Input: dimensioned drawing with shaded views. Units: mm. Origin: part minimum x, y, z. A direction names the side the tool comes from. Coordinates: 2 decimals unless noted, no trailing zeros. Loops run counter-clockwise (first coordinate to the right, second up) from the corner with the lowest first, then second, coordinate; pieces in that order, holes last. Notation, with made-up numbers: (-13, 32.5) - (36, 32.5) arc R17 cw to (36, 61.5) - close; hole circle Ø11 at (-16, 38.25). An arc over 180 degrees is marked (long way). Use one line per item in the form item = value. Start each with the question number.
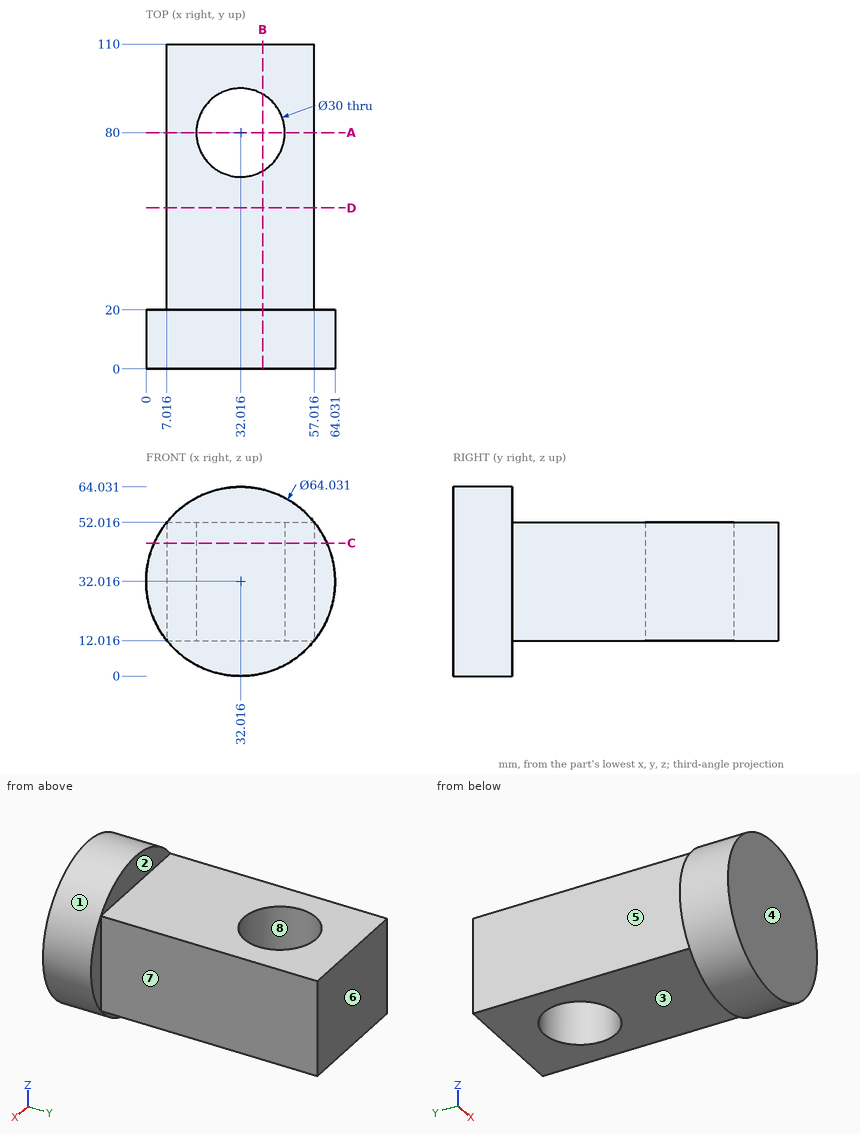
(1) Contact query for flat-ended pins moving along their axis: pin 1 (2 mm diameter, centred on x = 61, z = 38, fed in from +Y); pin 2 (20 mm diameter, centred on y = 64.5, z = 29, fed in from -X); pin 3 (2 mm diameter, centred on x = 45, y = 95, fed in from +Z); pin 4 (5 mm diameter, centred on y = 78.5, z = 9, fed in from -X). Output: stop coordinate, or through.
(2) Cut plane A-A, the plane y = 80. Output: boundary loops of the cut face in (x, z) (1 decimal), plus the area to 3 significant figures.
(3) Cut plane C-C, the plane z = 45. Output: boundary loops of the cut face in (x, y) (1 decimal), plus the area to 3 significant figures.
(4) Cut plane D-D, the plane y = 54.5. Output: boundary loops of the cut face in (x, z) (1 decimal), plus the area to 3 significant figures.
(5) Cut plane B-B, the plane x = 39.5. Output: boundary loops of the cut face in (y, z) (1 decimal).
(6) Access query for the marked faces 1, 2, 3, 4 and 5. Directions: +Z, -Z, +X, -X, +Y, -Y. A direction counts if a zero-diameter tool reaches every point of the face in a straight line with its end or side. Return the directions, or none.
(7) Material intervals for line 1 (Y direction, x = 18, z = 54.5); line 2 (Z direction, x = 52, y = 63) (1 decimal); line 3 (Y direction, x = 28, z = 21), sorted ascending.
(8) Mould query, pull axis Y, two halves, no side actions, for the marked faces 6, 7 and 8. Classes: +Y half, -Y half, draft (parallel to the pull), parting line (faces both ways), or undercut.
Recorded:
q1.pin_1 = 20
q1.pin_2 = 7.02
q1.pin_3 = 52.02
q1.pin_4 = through
q2.outline = (7, 12) - (17, 12) - (17, 52) - (7, 52) - close; (47, 12) - (57, 12) - (57, 52) - (47, 52) - close
q2.area = 800 mm²
q3.outline = (2.8, 0) - (61.3, 0) - (61.3, 20) - (57, 20) - (57, 110) - (7, 110) - (7, 20) - (2.8, 20) - close; hole circle Ø30 at (32, 80)
q3.area = 4,960 mm²
q4.outline = (7, 12) - (57, 12) - (57, 52) - (7, 52) - close
q4.area = 2,000 mm²
q5.outline = (0, 0.9) - (20, 0.9) - (20, 12) - (67, 12) - (67, 52) - (20, 52) - (20, 63.1) - (0, 63.1) - close; (93, 12) - (110, 12) - (110, 52) - (93, 52) - close
q6.face_1 = +Y, -Y
q6.face_2 = +Z, +X, -X, +Y
q6.face_3 = -Z, +X, -X, +Y
q6.face_4 = +Z, -Z, +X, -X, -Y
q6.face_5 = +Z, -Z, -X, +Y
q7.line_1 = 0 to 20
q7.line_2 = 12 to 52
q7.line_3 = 0 to 65.55, 94.45 to 110
q8.face_6 = +Y half
q8.face_7 = draft
q8.face_8 = undercut
